from build123d import *

# Parameters (mm, degrees)
SKETCH1_R           = 25
BOSS_EXTRUDE1_DEPTH = 10
SKETCH2_W           = 5
SKETCH2_H           = 30
BOSS_EXTRUDE2_DEPTH = 40
SKETCH3_R           = 2.5
CUT_EXTRUDE1_DEPTH  = 72.763500472


with BuildPart() as part:
    # Sketch1 → Boss-Extrude1 (new body)
    with BuildSketch(Plane(origin=(0, 0, 0), x_dir=(1, 0, 0), z_dir=(0, 1, 0))):
        with Locations(Location((0, 0, 0), (0, 0, 270))):
            Circle(SKETCH1_R)
    extrude(amount=BOSS_EXTRUDE1_DEPTH)

    # Sketch2 → Boss-Extrude2 (add)
    with BuildSketch(Plane(origin=(0, 10, 0), x_dir=(1, 0, 0), z_dir=(0, 1, 0))):
        with Locations((17.5, 0)):
            Rectangle(SKETCH2_W, SKETCH2_H)
        with Locations((-17.5, 0)):
            Rectangle(SKETCH2_W, SKETCH2_H)
    extrude(amount=BOSS_EXTRUDE2_DEPTH)

    # Sketch3 → Cut-Extrude1 (cut, through all)
    with BuildSketch(Plane.ZY.offset(20)):
        with BuildLine():
            Line((-15, 50), (-15, 30))
            ThreePointArc((-15, 30), (0, 45), (15, 30))
            Line((15, 30), (15, 50))
            Line((15, 50), (-15, 50))
        make_face()
        with Locations((0, 30)):
            Circle(SKETCH3_R)
    extrude(amount=-CUT_EXTRUDE1_DEPTH, mode=Mode.SUBTRACT)


solid = part.part
The listing builds one solid part. Answer for the finished solid, in the listing's coordinates (mm). A direction names the side the tool comes from. Give positions to 0.01 mm unless a question says otherwise; leave off trailing zeros. Order: outer loops, then holes, each group sorted by start corner. A loop starts at its lowest first (then second) coordinate and runs counter-clockwise, first axis right, second up. Notation, with made-up numbers: (-23.5, -15.5) -> (30.5, -15.5) arc R18 ccw to (30.5, -5.5) -> close; hole circle Ø9 at (-10.5, 6.5). An arc over 180 degrees is marked (long way). Put each result on its own line as item: value.
Item 1: A cutting plane is placed at B-B on y = 15.5. Give the vertices of the cut face in (x, z).
Established:
outline: (-20, -15) -> (-15, -15) -> (-15, 15) -> (-20, 15) -> close; (15, -15) -> (20, -15) -> (20, 15) -> (15, 15) -> close
Item 2: A cutting plane is placed at A-A on z = 0. Give the vertices of the cut face in (x, y).
Established:
outline: (-25, 0) -> (25, 0) -> (25, 10) -> (20, 10) -> (20, 27.5) -> (15, 27.5) -> (15, 10) -> (-15, 10) -> (-15, 27.5) -> (-20, 27.5) -> (-20, 10) -> (-25, 10) -> close; (-20, 32.5) -> (-15, 32.5) -> (-15, 45) -> (-20, 45) -> close; (15, 32.5) -> (20, 32.5) -> (20, 45) -> (15, 45) -> close
Item 3: For a pull along Z with two mould halves and no side action, classify faces 6 (the face through (17, 45, 0)), 7 (the face through (-18, 20, -15)), 8 (the face through (-17.54, 32.11, 1.34)) as released by +Z, released by -Z, zero draft, split by the parting line, or undercut.
Established:
face 6: split by the parting line
face 7: released by -Z
face 8: undercut
Item 4: For faces 1 (the face through (15, 27, 0)), 2 (the face through (17, 20, -15)), 3 (the face through (-20, 27, 0)), 4 (the face through (22, 10, 0)), 5 (the face through (17, 20, 15)), determine the directions among +Z, -Z, +X, -X, +Y, -Y from which every point of the face is accessible in a straight line to the end or side of a thin tool.
Established:
face 1: +Z, -Z, +Y
face 2: -Z, +X, -X, +Y
face 3: +Z, -Z, -X, +Y
face 4: +Z, -Z, +X, +Y
face 5: +Z, +X, -X, +Y
Item 5: A cutting plane is placed at D-D on z = -10.5. Give the vertices of the cut face in (x, y), plus the area to 3 significant figures.
Established:
outline: (-22.69, 0) -> (22.69, 0) -> (22.69, 10) -> (20, 10) -> (20, 40.71) -> (15, 40.71) -> (15, 10) -> (-15, 10) -> (-15, 40.71) -> (-20, 40.71) -> (-20, 10) -> (-22.69, 10) -> close
area: 761 mm^2
Item 6: Given P1, Ø15, axis at y = 20.5, z = -1, coming from the -X side; P2, Ø4, axis at x = 16.5, y = 16.5, coming from the +Z side; P3, Ø8, axis at x = 6.5, z = 5, coming from the -Y side; P4, Ø3, axis at y = 23.5, z = -11, coming from the +X side, each flat-ended and moving along its own axis, determine where each tip first touches the part or whether it passes through.
Established:
P1: stops at x = -20
P2: stops at z = 15
P3: stops at y = 0
P4: stops at x = 20
Item 7: A cutting plane is placed at C-C on y = 29. Give the vertices of the cut face in (x, z).
Established:
outline: (-20, -15) -> (-15, -15) -> (-15, -2.29) -> (-20, -2.29) -> close; (-20, 2.29) -> (-15, 2.29) -> (-15, 15) -> (-20, 15) -> close; (15, -15) -> (20, -15) -> (20, -2.29) -> (15, -2.29) -> close; (15, 2.29) -> (20, 2.29) -> (20, 15) -> (15, 15) -> close
Item 8: Straight lines are drawn through the part: line 1 (X direction, y = 25.5, z = -11); line 2 (Y direction, x = -18.05, z = 0); line 3 (Y direction, x = 8, z = -20). For each, find the intervals that lie inside material, in ascending order.
Established:
line 1: x = -20 to -15, 15 to 20
line 2: y = 0 to 27.5, 32.5 to 45
line 3: y = 0 to 10
